The model under review builds one solid part; all positions refer to its coordinate system, in mm. A direction names the side the tool comes from. Coordinates: 2 decimals unless noted, no trailing zeros. Write each loop counter-clockwise with the first axis right and the second up, starting at its lowest first coordinate (ties: lowest second). Pieces come first, ordered by that corner, then holes. Notation, with made-up numbers: (41, 23.5) - (98, 23.5) arc R22 cw to (98, 62.5) - close; hole circle Ø9 at (21.5, 7). An arc over 180 degrees is marked (long way). Put each result on its own line as item: value. Start each with the question number.
Item 1: Consider section A-A on x = 25. Give the boundary of the cut face in (y, z), then the cut area to 3 significant figures.
Item 2: Consider section D-D on x = 243.5. Give the boundary of the cut face in (y, z).
Item 3: Consider section B-B on z = 225. State how many separate pieces and enclosed holes the cut face has, then the cut area to 3 significant figures.
Item 4: For pin 1 (2 mm diameter, centred on y = 6, z = 87.5, fed in from -X); pin 2 (1 mm diameter, centred on y = 10, z = 31, fed in from -X); pin 3 (5 mm diameter, centred on x = 31.5, z = 102, fed in from +Y), all flat-tipped, find the tip position at first contact; note any pin that passes through.
Item 5: To check wall thickness, follow L1, parallel to Z at x = 25, y = 1.75; L2, parallel to Z at x = 150, y = 23; L3, parallel to X at y = 2.25, z = 225. State the ranges of each line that lie inside material, in increasing order. Write a range as [from, to].
Item 6: Mouldability with a two-part tool opening along Z and no side actions: class faces 1 (the face through (295, 1, 245)), 2 (the face through (269.755, 1.521, 24.769)), 3 (the face through (150, 25, 123)), 4 (the face through (159.237, 23.521, 228.83)) as pulls with the +Z half, pulls with the -Z half, needs draft (parallel to the pull), parting line crosses it, or undercut.
Item 7: Machinability: for faces 5 (the face through (49, 3, 123)), 6 (the face through (111, 11, 123)), 7 (the face through (149, 23, 250)), 8 (the face through (252, 3, 123)), which of the approach directions +Z, -Z, +X, -X, +Y, -Y give a long, thin tool a straight path to every point of the face, cutting with its end or side? Answer none if there is none.
Item 8: Consider section C-C on x = 150. Give the boundary of the cut face in (y, z).
```python
from build123d import *

# Parameters (mm, degrees)
EXTRUDE_1_DEPTH           = 250
HOLE_WIZARD_3_0_3_1_D     = 20
HOLE_WIZARD_3_0_3_1_DEPTH = 42.5
HOLE_WIZARD_3_0_3_1_TIP   = 6.00860619
FILLET_1_R                = 3
HOLE_WIZARD_10_5_10_5_1_D = 10.5
CHAMFER_1_SIZE            = 10


with BuildPart() as part:
    # 草图1 → 凸台-拉伸1 (new body)
    with BuildSketch(Plane.XY):
        Polygon((0, 0), (100, 0), (122, 22), (178, 22), (200, 0), (300, 0), (300, 3), (201.242640687, 3), (179.242640687, 25), (120.757359313, 25), (98.757359313, 3), (0, 3), align=None)
    extrude(amount=EXTRUDE_1_DEPTH)

    # Ø3.0 (3) 直径孔1
    with Locations(Plane(origin=(0, 22, 0), x_dir=(-1, 0, 0), z_dir=(0, -1, 0))):
        with Locations((-150, -225), (-150, -25)):
            Hole(HOLE_WIZARD_3_0_3_1_D / 2, depth=HOLE_WIZARD_3_0_3_1_DEPTH)
            with Locations((0, 0, -(HOLE_WIZARD_3_0_3_1_DEPTH + HOLE_WIZARD_3_0_3_1_TIP / 2))):  # 118° drill point
                Cone(0, HOLE_WIZARD_3_0_3_1_D / 2, HOLE_WIZARD_3_0_3_1_TIP, mode=Mode.SUBTRACT)

    # 圆角1
    fillet_1_edges = [part.edges().sort_by_distance(p)[0] for p in [
        (98.757359313, 3, 125),
        (120.757359313, 25, 125),
        (179.242640687, 25, 125),
        (201.242640687, 3, 125),
        (200, 0, 125),
        (178, 22, 125),
        (122, 22, 125),
        (100, 0, 125),
    ]]
    fillet(fillet_1_edges, radius=FILLET_1_R)

    # Ø10.5 (10.5) 直径孔1 (through all)
    with Locations(Plane(origin=(0, 0, 0), x_dir=(-1, 0, 0), z_dir=(0, -1, 0))):
        with Locations((-25, -225), (-25, -25), (-275, -225), (-275, -25)):
            Hole(HOLE_WIZARD_10_5_10_5_1_D / 2)

    # 倒角1
    chamfer_1_edges = [part.edges().sort_by_distance(p)[0] for p in [
        (300, 1.5, 0),
        (0, 1.5, 0),
        (300, 1.5, 250),
        (0, 1.5, 250),
    ]]
    chamfer(chamfer_1_edges, length=CHAMFER_1_SIZE)


solid = part.part
```
Report:
1. outline: (0, 0) - (3, 0) - (3, 19.75) - (0, 19.75) - close; (0, 30.25) - (3, 30.25) - (3, 219.75) - (0, 219.75) - close; (0, 230.25) - (3, 230.25) - (3, 250) - (0, 250) - close
1. area: 687 mm²
2. outline: (0, 0) - (3, 0) - (3, 250) - (0, 250) - close
3. separate pieces: 4
3. enclosed holes: 0
3. area: 832 mm²
4. pin 1: x = 100.76
4. pin 2: x = 105.26
4. pin 3: y = 3
5. L1: [0, 19.75], [30.25, 219.75], [230.25, 250]
5. L2: [0, 15], [35, 215], [235, 250]
5. L3: [0, 19.75], [30.25, 102.25], [197.75, 269.75], [280.25, 300]
6. face 1: pulls with the +Z half
6. face 2: undercut
6. face 3: needs draft
6. face 4: undercut
7. face 5: +Z, -Z, -X, +Y
7. face 6: +Z, -Z, -Y
7. face 7: +Z, +X, -X, +Y, -Y
7. face 8: +Z, -Z, +X, +Y
8. outline: (22, 0) - (25, 0) - (25, 15) - (22, 15) - close; (22, 35) - (25, 35) - (25, 215) - (22, 215) - close; (22, 235) - (25, 235) - (25, 250) - (22, 250) - close
